from build123d import *

# Parameters (mm, degrees)
ESQUISSE1_W           = 3.85
ESQUISSE1_H           = 6.2
ESQUISSE1_R           = 1.25
PLAQUE_DEPTH          = 0.5
CORPS_DEPTH           = 6.85
CONG_R                = 0.5
ESQUISSE2_W           = 9.2
ESQUISSE2_H           = 4.25
CAVIT_DEPTH           = 1
ESQUISSE3_W           = 5.5
ESQUISSE3_H           = 3.75
BOUTON_DEPTH          = 10.2
RELIEF_DEPTH          = 16.856958252
CONG_2_R              = 0.4
ESQUISSE6_W           = 2.15
ESQUISSE6_H           = 0.38
PIN_DEPTH             = 4.4
ARRONDI_DEPTH         = 0.38
PERCAGE_DEPTH         = 0.38
R_P_TITION_COUNT      = 3
R_P_TITION_PITCH      = 3.925
R_P_TITION_COUNT_DIR2 = 2
R_P_TITION_PITCH_DIR2 = 2.52


with BuildPart() as part:
    # Esquisse1 → Plaque (new body)
    # profile 1 of 2: a face of its own
    with BuildSketch(Plane(origin=(0, 0, 0), x_dir=(1, 0, 0), z_dir=(0, 1, 0))):
        with Locations((-9.725, 0)):
            Rectangle(ESQUISSE1_W, ESQUISSE1_H)
        with Locations(Location((-9.4, 0, 0), (0, 0, 270))):
            Circle(ESQUISSE1_R, mode=Mode.SUBTRACT)
    # profile 2 of 2: a face of its own
    with BuildSketch(Plane(origin=(0, 0, 0), x_dir=(1, 0, 0), z_dir=(0, 1, 0))):
        with Locations((9.725, 0)):
            Rectangle(ESQUISSE1_W, ESQUISSE1_H)
        with Locations(Location((9.4, 0, 0), (0, 0, 270))):
            Circle(ESQUISSE1_R, mode=Mode.SUBTRACT)
    extrude(amount=-PLAQUE_DEPTH)

    # Esquisse1<5> → Corps (add)
    with BuildSketch(Plane(origin=(0, 0, 0), x_dir=(1, 0, 0), z_dir=(0, 1, 0))):
        Polygon((7.8, 3.1), (7.8, -3.1), (7.8, -3.7), (-7.8, -3.7), (-7.8, -3.1), (-7.8, 3.1), (-7.8, 3.7), (7.8, 3.7), align=None)
    extrude(amount=-CORPS_DEPTH)

    # Congé
    cong_edges = [part.edges().sort_by_distance(p)[0] for p in [
        (-11.65, -0.25, 3.1),
        (-11.65, -0.25, -3.1),
        (11.65, -0.25, -3.1),
        (11.65, -0.25, 3.1),
    ]]
    fillet(cong_edges, radius=CONG_R)

    # Esquisse2 → Cavité (cut)
    with BuildSketch(Plane(origin=(0, 0, 0), x_dir=(1, 0, 0), z_dir=(0, 1, 0))):
        Rectangle(ESQUISSE2_W, ESQUISSE2_H)
    extrude(amount=-CAVIT_DEPTH, mode=Mode.SUBTRACT)

    # Esquisse3 → Bouton (add)
    with BuildSketch(Plane(origin=(0, -1, 0), x_dir=(1, 0, 0), z_dir=(0, 1, 0))):
        with Locations((-1.85, 0)):
            Rectangle(ESQUISSE3_W, ESQUISSE3_H)
    extrude(amount=BOUTON_DEPTH)

    # Esquisse5 → Relief (cut, through all)
    with BuildSketch(Plane.XY.offset(1.875)):
        Polygon((-4.6, 9.2), (-4.6, 8.05), (-4.05, 8.75), (-3.5, 8.35), (-2.95, 9.05), (-2.4, 8.5), (-1.85, 9.2), align=None)
        Polygon((0.9, 9.2), (-1.85, 9.2), (-1.3, 8.5), (-0.75, 9.05), (-0.2, 8.35), (0.35, 8.75), (0.9, 8.05), align=None)
    extrude(amount=-RELIEF_DEPTH, mode=Mode.SUBTRACT)

    # Congé2
    cong_2_edges = [part.edges().sort_by_distance(p)[0] for p in [
        (0, 0, -3.7),
        (0, 0, 3.7),
    ]]
    fillet(cong_2_edges, radius=CONG_2_R)

    # Esquisse6 → Pin (add)
    with BuildSketch(Plane.XZ.offset(6.85)):
        with Locations((-3.925, 1.21)):
            Rectangle(ESQUISSE6_W, ESQUISSE6_H)
    pin = extrude(amount=PIN_DEPTH)

    # Esquisse8 → Arrondi (cut)
    with BuildSketch(Plane.XY.offset(1.4)):
        with BuildLine():
            Line((-4.8, -7.45), (-5, -7.15))
            Line((-5, -7.15), (-5, -11.25))
            Line((-5, -11.25), (-3.925, -11.25))
            ThreePointArc((-3.925, -11.25), (-4.543718434, -10.993718434), (-4.8, -10.375))
            Line((-4.8, -10.375), (-4.8, -7.45))
        make_face()
        with BuildLine():
            Line((-2.85, -11.25), (-2.85, -7.15))
            Line((-2.85, -7.15), (-3.05, -7.45))
            Line((-3.05, -7.45), (-3.05, -10.375))
            ThreePointArc((-3.05, -10.375), (-3.306281566, -10.993718434), (-3.925, -11.25))
            Line((-3.925, -11.25), (-2.85, -11.25))
        make_face()
    arrondi = extrude(amount=-ARRONDI_DEPTH, mode=Mode.SUBTRACT)

    # Esquisse9 → Percage (cut)
    with BuildSketch(Plane.XY.offset(1.4)):
        with BuildLine():
            Line((-4.425, -10.15), (-4.425, -9.55))
            ThreePointArc((-4.425, -9.55), (-3.925, -9.05), (-3.425, -9.55))
            Line((-3.425, -9.55), (-3.425, -10.15))
            ThreePointArc((-3.425, -10.15), (-3.925, -10.65), (-4.425, -10.15))
        make_face()
    percage = extrude(amount=-PERCAGE_DEPTH, mode=Mode.SUBTRACT)

    # Répétition: Pin, Arrondi, Percage 3 × 2
    with Locations(*[(i * R_P_TITION_PITCH, 0, -j * R_P_TITION_PITCH_DIR2) for i in range(R_P_TITION_COUNT) for j in range(R_P_TITION_COUNT_DIR2) if (i, j) != (0, 0)]):
        add(pin)
        add(arrondi, mode=Mode.SUBTRACT)
        add(percage, mode=Mode.SUBTRACT)


solid = part.part
Work out the finished part from the listing and answer in its coordinate system (mm). A direction names the side the tool comes from. Give positions to 0.01 mm unless a question says otherwise; leave off trailing zeros. Loops run counter-clockwise (first coordinate to the right, second up) from the corner with the lowest first, then second, coordinate; pieces in that order, holes last. Notation, with made-up numbers: (-14.75, -3) - (7.25, -3) arc R13 ccw to (7.25, 9) - close; hole circle Ø2 at (48.25, 88). An arc over 180 degrees is marked (long way). Answer in a Markdown table with one row per item. Add a question column.
Q1. The part is cut by section D-D (y = 6.5). Determine the outline of the cut face in (x, z) (3 decimals).
Q2. Consider line 1 along X through (y, z) = (-0.15, 0); line 2 along X through (y, z) = (-4.25, 2.25); line 3 along Y through (x, z) = (-9, -2.5). Determine where each line is inside the solid, lowest interval first.
Q3. A tool of negligible diameter and unlimited length cuts with its end or side. For faces 4 (the flat face through (0, -8.5, -1.5)), 5 (the flat face through (-11, -0.5, 1)), 6 (the flat face through (3.9, -8.5, -1.12)), 7 (the flat face through (4.6, -0.5, 0)), 8 (the flat face through (0, -8.5, 1.4)), from which of +Z, -Z, +X, -X, +Y, -Y can it reach the whole face along a straight path? Write none if from no direction.
Q4. The part is cut by section C-C (z = 0.75). State how many separate pieces and enclosed holes the cut face has, and give its area (3 significant figures).
Q5. Each of these flat-tipped pins is pushed along its axis until it touches: P1, Ø1.9, axis at x = 9.5, z = 0, coming from the -Y side (3 decimals); P2, Ø3, axis at x = -6.5, z = 1.5, coming from the +Y side; P3, Ø2, axis at x = -2, z = 0, coming from the +Y side; P4, Ø3, axis at y = 2.5, z = -1, coming from the +X side. Where does it stop, or does it pass through?
Q6. The part is cut by section A-A (y = -8). Determine the outline of the cut face in (x, z) (3 decimals).
Q7. Determine the mould class of faces 1 (the cylindrical face through (8.64, -0.25, -0.99)), 2 (the flat face through (0, -4, 3.7)), 3 (the flat face through (7.8, -3, 0)) for opening direction Z: released by +Z, released by -Z, zero draft, split by the parting line, or undercut.
Q8. The part is cut by section B-B (x = 9.75). Determine the outline of the cut face in (y, z).
Solution:
| question | item | result |
|---|---|---|
| 1 | outline | (-4.6, -1.875) - (0.9, -1.875) - (0.9, 1.875) - (-4.6, 1.875) - close |
| 2 | line 1 | x = -11.65 to -10.65, -8.15 to 0.9, 4.6 to 8.15, 10.65 to 11.65 |
| 2 | line 2 | x = -7.8 to 7.8 |
| 2 | line 3 | y = -0.5 to 0 |
| 3 | face 4 | -Z, +X, -X, -Y |
| 3 | face 5 | +Z, -Z, -X, -Y |
| 3 | face 6 | +X, -X, -Y |
| 3 | face 7 | +Y |
| 3 | face 8 | +Z, +X, -X, -Y |
| 4 | separate pieces | 3 |
| 4 | enclosed holes | 0 |
| 4 | area | 153 mm² |
| 5 | P1 | passes through |
| 5 | P2 | stops at y = 0 |
| 5 | P3 | stops at y = 9.2 |
| 5 | P4 | stops at x = 0.9 |
| 6 | outline | (-4.8, -1.5) - (-3.05, -1.5) - (-3.05, -1.12) - (-4.8, -1.12) - close; (-4.8, 1.02) - (-3.05, 1.02) - (-3.05, 1.4) - (-4.8, 1.4) - close; (-0.875, -1.5) - (0.875, -1.5) - (0.875, -1.12) - (-0.875, -1.12) - close; (-0.875, 1.02) - (0.875, 1.02) - (0.875, 1.4) - (-0.875, 1.4) - close; (3.05, -1.5) - (4.8, -1.5) - (4.8, -1.12) - (3.05, -1.12) - close; (3.05, 1.02) - (4.8, 1.02) - (4.8, 1.4) - (3.05, 1.4) - close |
| 7 | face 1 | undercut |
| 7 | face 2 | released by +Z |
| 7 | face 3 | zero draft |
| 8 | outline | (-0.5, -3.1) - (0, -3.1) - (0, -1.2) - (-0.5, -1.2) - close; (-0.5, 1.2) - (0, 1.2) - (0, 3.1) - (-0.5, 3.1) - close |
